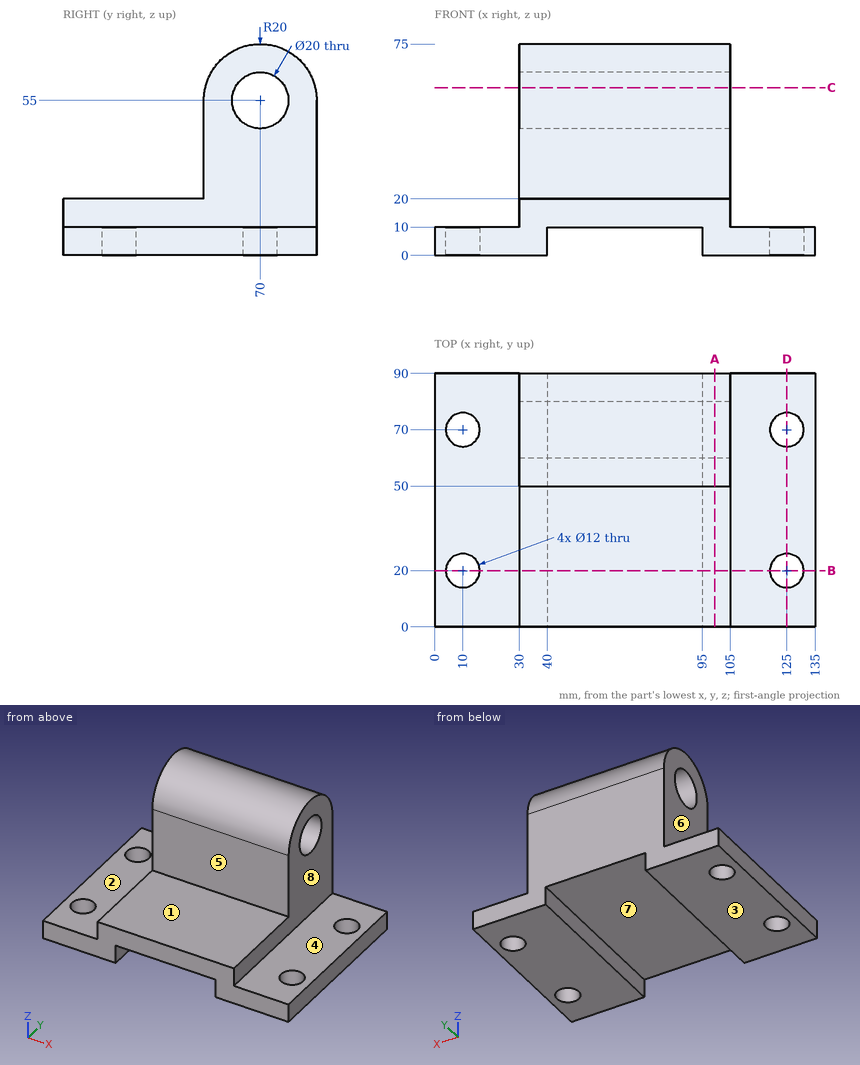
Answer from the drawing. Dimensions are ordinates in mm from the lowest x, y and z of the part. A direction names the side the tool comes from. Give positions to 0.01 mm unless a question says otherwise; leave off trailing zeros. Loops run counter-clockwise (first coordinate to the right, second up) from the corner with the lowest first, then second, coordinate; pieces in that order, holes last. Notation, with made-up numbers: (57.25, 6.25) -> (62.25, 6.25) arc R5 cw to (62.25, 15.25) -> close; hole circle Ø1 at (-12, 71). An arc over 180 degrees is marked (long way). Use a Markdown table: item, result.
Q1. Determine the mould class of the marked faces 5, 6, 7 and 8 for opening direction X: pulls with the +X half, pulls with the -X half, needs draft (parallel to the pull), parting line crosses it, or undercut.
Solved:
| item | result |
|---|---|
| face 5 | needs draft |
| face 6 | pulls with the -X half |
| face 7 | undercut |
| face 8 | pulls with the +X half |
Q2. Section A-A, the plane x = 99.5 is taken. Determine the outline of the cut face in (y, z).
Solved:
| item | result |
|---|---|
| outline | (0, 0) -> (90, 0) -> (90, 55) arc R20 ccw to (50, 55) -> (50, 20) -> (0, 20) -> close; hole circle Ø20 at (70, 55) |
Q3. A tool of negligible diameter and unlimited length cuts with its end or side. For the marked faces 1, 2, 3 and 4, from which of +Z, -Z, +X, -X, +Y, -Y can it reach the whole face along a straight path? Write none if from no direction.
Solved:
| item | result |
|---|---|
| face 1 | +Z, +X, -X, -Y |
| face 2 | +Z, -X, +Y, -Y |
| face 3 | -Z, +X, -X, +Y, -Y |
| face 4 | +Z, +X, +Y, -Y |
Q4. Section C-C, the plane z = 59.5 is taken. Determine the outline of the cut face in (x, y), then the cut area to 3 significant figures.
Solved:
| item | result |
|---|---|
| outline | (30, 50.51) -> (105, 50.51) -> (105, 61.07) -> (30, 61.07) -> close; (30, 78.93) -> (105, 78.93) -> (105, 89.49) -> (30, 89.49) -> close |
| area | 1,580 mm^2 |
Q5. Section B-B, the plane y = 20 is taken. Determine the outline of the cut face in (x, z).
Solved:
| item | result |
|---|---|
| outline | (0, 0) -> (4, 0) -> (4, 10) -> (0, 10) -> close; (16, 0) -> (40, 0) -> (40, 10) -> (95, 10) -> (95, 0) -> (119, 0) -> (119, 10) -> (105, 10) -> (105, 20) -> (30, 20) -> (30, 10) -> (16, 10) -> close; (131, 0) -> (135, 0) -> (135, 10) -> (131, 10) -> close |
Q6. Section D-D, the plane x = 125 is taken. Determine the outline of the cut face in (y, z), then the cut area to 3 significant figures.
Solved:
| item | result |
|---|---|
| outline | (0, 0) -> (14, 0) -> (14, 10) -> (0, 10) -> close; (26, 0) -> (64, 0) -> (64, 10) -> (26, 10) -> close; (76, 0) -> (90, 0) -> (90, 10) -> (76, 10) -> close |
| area | 660 mm^2 |
Q7. Each of these flat-tipped pins is pushed along its axis until it touches: pin 1 (9.5 mm diameter, centred on x = 10, y = 20, fed in from +Z); pin 2 (2 mm diameter, centred on x = 63, y = 9, fed in from -Z); pin 3 (15 mm diameter, centred on x = 22, y = 59.5, fed in from +Z); pin 4 (2 mm diameter, centred on x = 50, y = 60, fed in from +Z). Where does it stop, or does it pass through?
Solved:
| item | result |
|---|---|
| pin 1 | passes through |
| pin 2 | stops at z = 10 |
| pin 3 | stops at z = 10 |
| pin 4 | stops at z = 72.86 |
Q8. Find the intervals of material crossed by line 1 along Y through (x, z) = (125, 7); line 2 along Z through (x, y) = (83.5, 70); line 3 along Z through (x, y) = (13, 34), in increasing order.
Solved:
| item | result |
|---|---|
| line 1 | y = 0 to 14, 26 to 64, 76 to 90 |
| line 2 | z = 10 to 45, 65 to 75 |
| line 3 | z = 0 to 10 |
